```python
from build123d import *

# Parameters (mm, degrees)
SKETCH2_R           = 7
SKETCH2_R_2         = 0.58
BOSS_EXTRUDE1_DEPTH = 1
SKETCH3_R           = 3
SKETCH3_R_2         = 2.5
EXTRUDE_THIN1_DEPTH = 2


with BuildPart() as part:
    # Sketch2 → Boss-Extrude1 (new body)
    with BuildSketch(Plane.XY):
        Circle(SKETCH2_R)
        with Locations((4.27289846, 3.557518623)):
            Circle(SKETCH2_R_2, mode=Mode.SUBTRACT)
        with Locations((-4.27289846, 3.557518623)):
            Circle(SKETCH2_R_2, mode=Mode.SUBTRACT)
        with Locations((4.27289846, -3.557518623)):
            Circle(SKETCH2_R_2, mode=Mode.SUBTRACT)
        with Locations((-4.27289846, -3.557518623)):
            Circle(SKETCH2_R_2, mode=Mode.SUBTRACT)
    extrude(amount=BOSS_EXTRUDE1_DEPTH)

    # Sketch3 → Extrude-Thin1 (add)
    with BuildSketch(Plane.XY.offset(1)):
        Circle(SKETCH3_R)
        Circle(SKETCH3_R_2, mode=Mode.SUBTRACT)
    extrude(amount=EXTRUDE_THIN1_DEPTH)


solid = part.part
```
Check sheet for the modelled part. Datum: model origin and axes. Units: mm. A direction names the side the tool comes from. Round coordinates to 2 decimals unless told otherwise and drop trailing zeros. Loops run counter-clockwise (first coordinate to the right, second up) from the corner with the lowest first, then second, coordinate; pieces in that order, holes last. Notation, with made-up numbers: (69, -29) - (84, -29) arc R25 cw to (84, 10) - close; hole circle Ø9 at (-24, 52). An arc over 180 degrees is marked (long way). Answer as a JSON object with one key per item and string values. Group by question number.
Q1. Set-up check for faces 4 (the face through (-3.737, -3.78, 0.493)), 5 (the face through (0, 0, 1)): record each of +Z, -Z, +X, -X, +Y, -Y from which the full face is reachable in a straight line by a thin tool's end or side.
Q2. Mould release check, pull along X, two halves, no side actions. Record for faces 1 (the face through (4.15, 2.99, 0.49)), 2 (the face through (1, -3, 1)), 3 (the face through (6.466, -2.681, 0.493)): released by +X, released by -X, zero draft, split by the parting line, or undercut.
Q3. Gauge pin test, flat end, axial feed: P1, Ø6, axis at x = 0, y = 0, coming from the +Z side. Record the tip position at first contact, or that the pin passes through.
Q4. Sectioned sample at A-A, the plane x = 0. Enter the section's corners in (y, z).
Q5. Sectioned sample at C-C, the plane z = 1.9. Enter the section's corners in (x, y), plus the area to 3 significant figures.
Q6. Scan lines: line 1 along Y through (x, z) = (0, 1.7); line 2 along Y through (x, z) = (4.25, 0.3); line 3 along Z through (x, y) = (-2, -1). Record each from-to range of solid material in increasing order. Write a range as [from, to].
Q7. Sectioned sample at D-D, the plane y = -4.5. Enter the section's corners in (x, z), plus the area to 3 significant figures.
Solution:
{
 "1": {"face 4": "+Z, -Z", "face 5": "+Z"},
 "2": {"face 1": "undercut", "face 2": "zero draft", "face 3": "split by the parting line"},
 "3": {"P1": "stops at z = 3"},
 "4": {"outline": "(-7, 0) - (7, 0) - (7, 1) - (3, 1) - (3, 3) - (2.5, 3) - (2.5, 1) - (-2.5, 1) - (-2.5, 3) - (-3, 3) - (-3, 1) - (-7, 1) - close"},
 "5": {"outline": "circle Ø6 at (0, 0); hole circle Ø5 at (0, 0)", "area": "8.64 mm²"},
 "6": {"line 1": "y = [-3, -2.5], [2.5, 3]", "line 2": "y = [-5.56, -4.14], [-2.98, 2.98], [4.14, 5.56]", "line 3": "z = [0, 1]"},
 "7": {"outline": "(-5.36, 0) - (5.36, 0) - (5.36, 1) - (-5.36, 1) - close", "area": "10.7 mm²"}
}
